Geometry check sheet. Reference: drawing and pictorial views, mm from the part's lowest x, y, z. A direction names the side the tool comes from. Round coordinates to 2 decimals unless told otherwise and drop trailing zeros. Loops run counter-clockwise (first coordinate to the right, second up) from the corner with the lowest first, then second, coordinate; pieces in that order, holes last. Notation, with made-up numbers: (33.25, -15) - (72.25, -15) arc R19 cw to (72.25, 16) - close; hole circle Ø5 at (-5, 22). An arc over 180 degrees is marked (long way). Return JSON: item names as keys, results as strings.
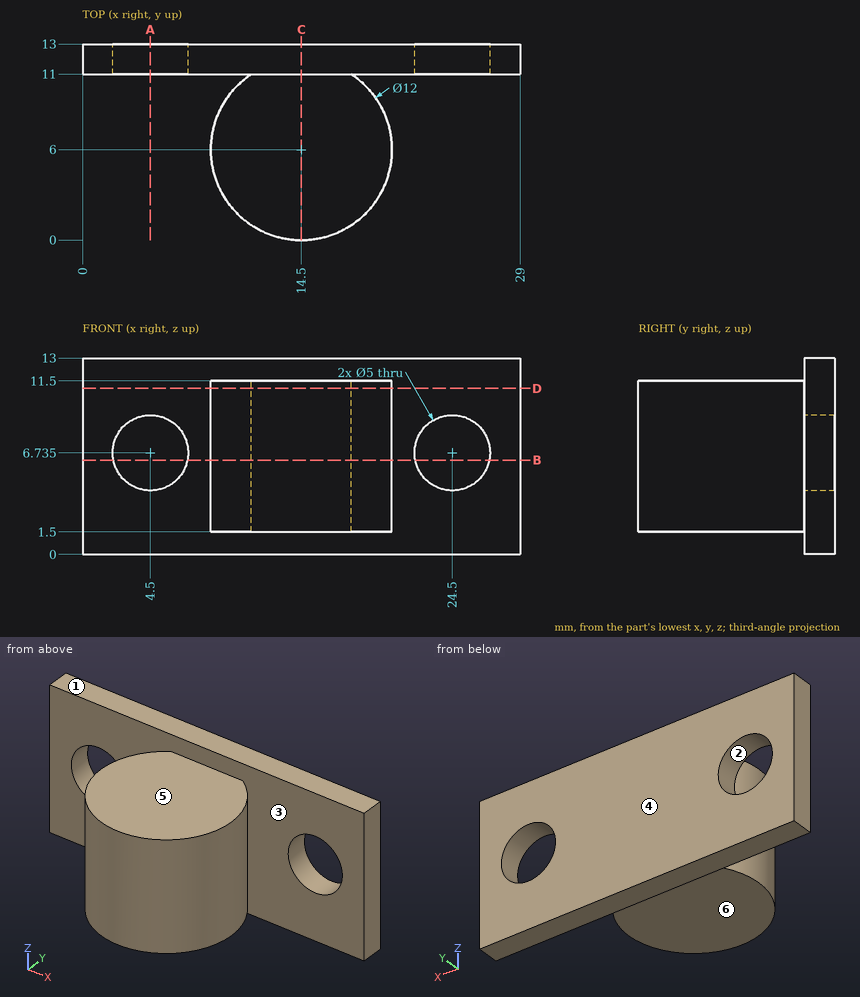
Q1. Draft check along Z on the marked faces 1, 2 and 3. Enter one of: released by +Z, released by -Z, zero draft, split by the parting line, or undercut.
Answer key:
{"face 1": "released by +Z", "face 2": "undercut", "face 3": "zero draft"}
Q2. Depth check by flat-ended pin: P1, Ø5, axis at y = 7, z = 4.5, coming from the -X side; P2, Ø4.5, axis at x = 4.5, z = 6.73, coming from the +Y side. Enter the tip coordinate at first touch or a pass-through.
Answer key:
{"P1": "stops at x = 8.5", "P2": "passes through"}
Q3. Sectioned sample at B-B (z = 6.25). Enter the section's corners in (x, y), plus the area to 3 significant figures.
Answer key:
{"outline": "(0, 11) - (2.05, 11) - (2.05, 13) - (0, 13) - close; (6.95, 11) - (11.18, 11) arc R6 ccw (long way) to (17.82, 11) - (22.05, 11) - (22.05, 13) - (6.95, 13) - close; (26.95, 11) - (29, 11) - (29, 13) - (26.95, 13) - close", "area": "147 mm²"}
Q4. Scan lines: probe 1 along Z at (x, y) = (24.5, 12.1) (3 decimals); probe 2 along Z at (x, y) = (12.75, 6.5); probe 3 along Y at (x, z) = (22.25, 4.75). Record each from-to range of solid material in increasing order. Write a range as [from, to].
Answer key:
{"probe 1": "z = [0, 4.235], [9.235, 13]", "probe 2": "z = [1.5, 11.5]", "probe 3": "y = [11, 13]"}
Q5. Sectioned sample at A-A (x = 4.5). Enter the section's corners in (y, z) (3 decimals), plus the area to 3 significant figures.
Answer key:
{"outline": "(11, 0) - (13, 0) - (13, 4.235) - (11, 4.235) - close; (11, 9.235) - (13, 9.235) - (13, 13) - (11, 13) - close", "area": "16.0 mm²"}
Q6. Sectioned sample at D-D (z = 11). Enter the section's corners in (x, y), plus the area to 3 significant figures.
Answer key:
{"outline": "(0, 11) - (11.18, 11) arc R6 ccw (long way) to (17.82, 11) - (29, 11) - (29, 13) - (0, 13) - close", "area": "167 mm²"}
Q7. Tool access check on the marked faces 4, 5 and 6. Record the directions out of +Z, -Z, +X, -X, +Y, -Y that give a thin tool (end or side, any length) a straight path to the whole face; none if there is none.
Answer key:
{"face 4": "+Z, -Z, +X, -X, +Y", "face 5": "+Z, +X, -X, -Y", "face 6": "-Z, +X, -X, -Y"}
Q8. Sectioned sample at C-C (x = 14.5). Enter the section's corners in (y, z).
Answer key:
{"outline": "(0, 1.5) - (11, 1.5) - (11, 0) - (13, 0) - (13, 13) - (11, 13) - (11, 11.5) - (0, 11.5) - close"}
